The figure shows three views and two pictorial views of one solid part (mm, origin at its lowest corner). Answer the questions. A direction names the side the tool comes from. Coordinates: 2 decimals unless noted, no trailing zeros. Loops run counter-clockwise (first coordinate to the right, second up) from the corner with the lowest first, then second, coordinate; pieces in that order, holes last.
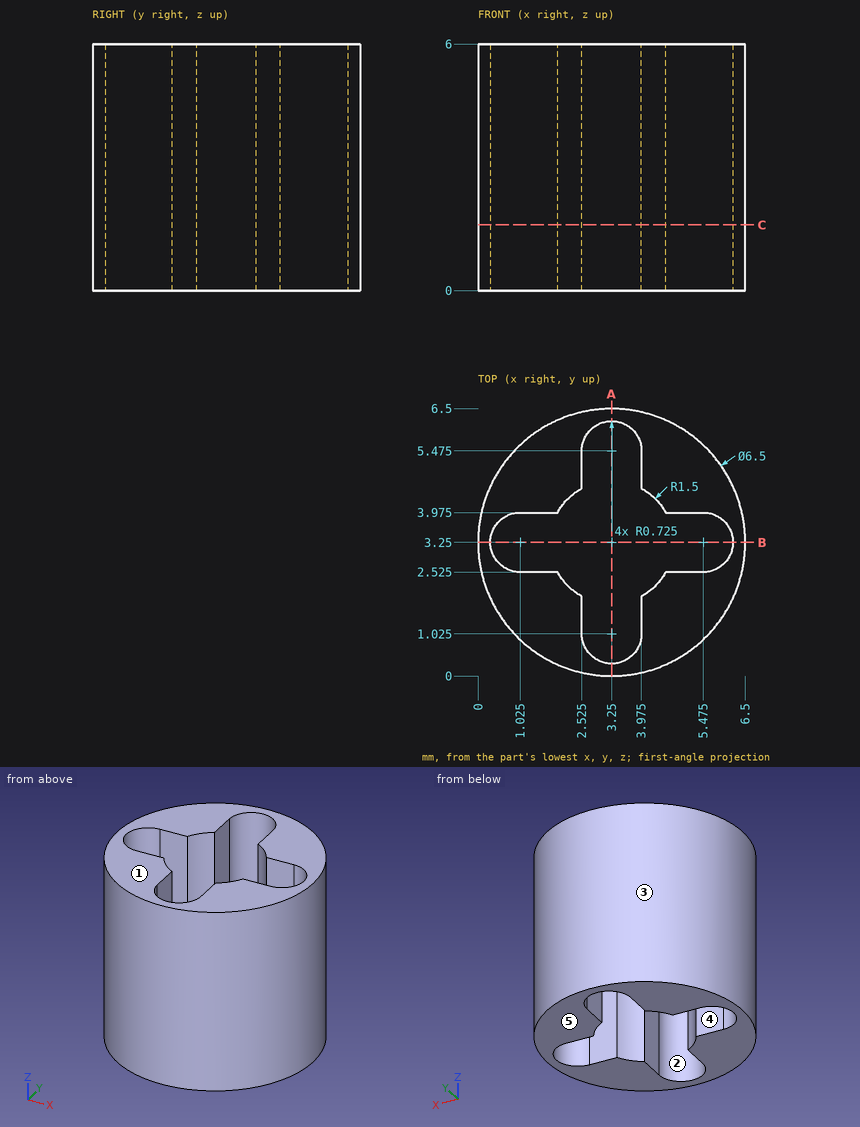
Q1. Which of the six approach directions +Z, -Z, +X, -X, +Y, -Y give full straight-line access (tool end or side, diameter ignored) to the marked faces 4 and 5?
Findings below:
face 4: +Z, -Z
face 5: -Z, +X, -X, +Y, -Y
Q2. A cutting plane is placed at A-A (x = 3.25). Give the vertices of the cut face in (y, z).
Findings below:
outline: (0, 0) - (0.3, 0) - (0.3, 6) - (0, 6) - close; (6.2, 0) - (6.5, 0) - (6.5, 6) - (6.2, 6) - close
Q3. Straight lines are drawn through the part: probe 1 along X at (y, z) = (3.5, 0.4); probe 2 along Y at (x, z) = (2, 0.35); probe 3 along X at (y, z) = (1.75, 4.1) (3 decimals). For each, find the intervals that lie inside material, in ascending order.
Findings below:
probe 1: x = 0.01 to 0.34, 6.16 to 6.49
probe 2: y = 0.25 to 2.42, 4.08 to 6.25
probe 3: x = 0.367 to 2.525, 3.975 to 6.133
Q4. A cutting plane is placed at C-C (z = 1.6). Give the vertices of the cut face in (x, y) (3 decimals).
Findings below:
outline: circle Ø6.5 at (3.25, 3.25); hole (1.025, 2.525) - (1.937, 2.525) arc R1.5 ccw to (2.525, 1.937) - (2.525, 1.025) arc R0.725 ccw to (3.975, 1.025) - (3.975, 1.937) arc R1.5 ccw to (4.563, 2.525) - (5.475, 2.525) arc R0.725 ccw to (5.475, 3.975) - (4.563, 3.975) arc R1.5 ccw to (3.975, 4.563) - (3.975, 5.475) arc R0.725 ccw to (2.525, 5.475) - (2.525, 4.563) arc R1.5 ccw to (1.937, 3.975) - (1.025, 3.975) arc R0.725 ccw to start
Q5. Flat-ended cylindrical pins translate along their axes: pin 1 Ø0.5 at (x, z) = (1.5, 2.5) entering from -Y; pin 2 Ø3 at (x, z) = (1.5, 2) entering from +Y; pin 3 Ø1 at (y, z) = (5.5, 2) entering from +X; pin 4 Ø1 at (x, z) = (3.5, 5) entering from -Y. Find the tip coordinate at first contact, or state that the pin passes through.
Findings below:
pin 1: stops at y = 0.37
pin 2: stops at y = 6.49
pin 3: stops at x = 5.99
pin 4: stops at y = 0
Q6. Determine the mould class of the marked faces 1, 2 and 3 for opening direction X: +X half, -X half, draft (parallel to the pull), parting line (faces both ways), or undercut.
Findings below:
face 1: draft
face 2: undercut
face 3: parting line
